Check sheet for the drawn part. Datum: minimum x, y, z corner. Units: mm. Give positions to 0.01 mm unless a question says otherwise; leave off trailing zeros. Loops run counter-clockwise (first coordinate to the right, second up) from the corner with the lowest first, then second, coordinate; pieces in that order, holes last.
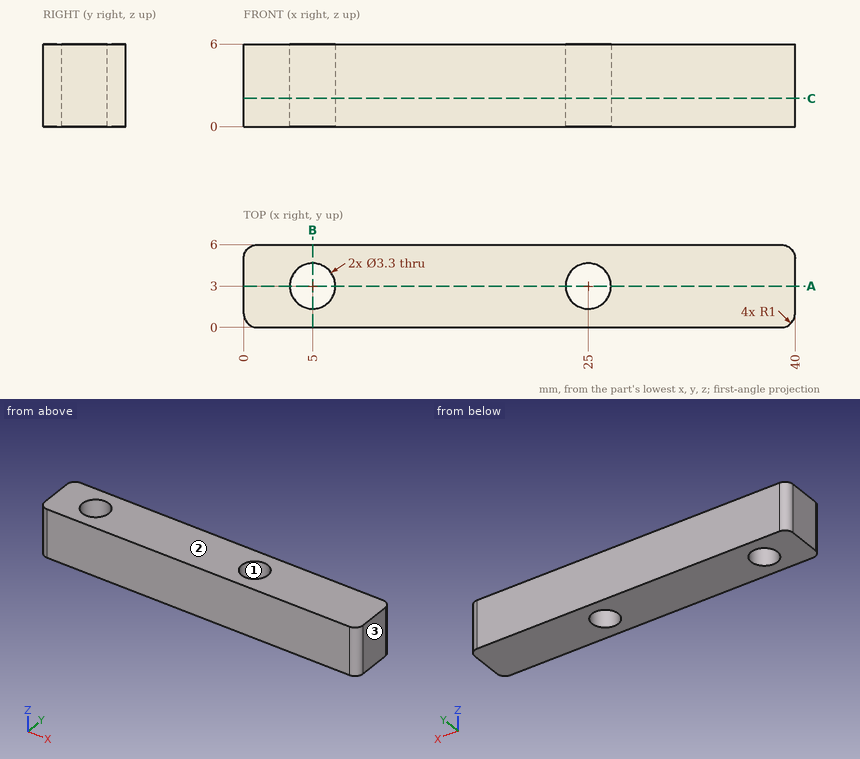
(1) Section check C-C on z = 2.05. Record the boundary of the cut face in (x, y), plus the area to 3 significant figures.
(2) Section check A-A on y = 3. Record the boundary of the cut face in (x, z).
(3) Section check B-B on x = 5. Record the boundary of the cut face in (y, z), plus the area to 3 significant figures.
(4) Material ranges on line 1 (Y direction, x = 25, z = 4.35); line 2 (X direction, y = 4.4, z = 5.15); line 3 (X direction, y = 3.9, z = 2), recorded low to high.
(5) Release check for a two-part mould opening along X. For the marked faces 1, 2 and 3 record: pulls with the +X half, pulls with the -X half, needs draft (parallel to the pull), parting line crosses it, or undercut.
(6) Gauge pin test, flat end, axial feed: pin 1 Ø3 at (x, y) = (25, 3) entering from +Z. Record the tip position at first contact, or that the pin passes through.
Computed values:
1. outline: (0, 1) arc R1 ccw to (1, 0) - (39, 0) arc R1 ccw to (40, 1) - (40, 5) arc R1 ccw to (39, 6) - (1, 6) arc R1 ccw to (0, 5) - close; hole circle Ø3.3 at (5, 3); hole circle Ø3.3 at (25, 3)
1. area: 222 mm2
2. outline: (0, 0) - (3.35, 0) - (3.35, 6) - (0, 6) - close; (6.65, 0) - (23.35, 0) - (23.35, 6) - (6.65, 6) - close; (26.65, 0) - (40, 0) - (40, 6) - (26.65, 6) - close
3. outline: (0, 0) - (1.35, 0) - (1.35, 6) - (0, 6) - close; (4.65, 0) - (6, 0) - (6, 6) - (4.65, 6) - close
3. area: 16.2 mm2
4. line 1: y = 0 to 1.35, 4.65 to 6
4. line 2: x = 0 to 4.13, 5.87 to 24.13, 25.87 to 40
4. line 3: x = 0 to 3.62, 6.38 to 23.62, 26.38 to 40
5. face 1: undercut
5. face 2: needs draft
5. face 3: pulls with the +X half
6. pin 1: passes through
